Check sheet for the modelled part. Datum: model origin and axes. Units: mm. A direction names the side the tool comes from. Give positions to 0.01 mm unless a question says otherwise; leave off trailing zeros. Order: outer loops, then holes, each group sorted by start corner. A loop starts at its lowest first (then second) coordinate and runs counter-clockwise, first axis right, second up. Notation, with made-up numbers: (-7, 47.25) -> (41, 47.25) arc R24 ccw to (41, 83.25) -> close; hole circle Ø5 at (-33, -30.5). An arc over 180 degrees is marked (long way). One line per question, with ' | ' between items.
```python
from build123d import *

# Parameters (mm, degrees)
IZIM1_W                     = 20
IZIM1_H                     = 20
Y_KSEKLIK_EKSTR_ZYON1_DEPTH = 20
KES_EKSTR_ZYON1_DEPTH       = 20
IZIM3_W                     = 17.224679165
IZIM3_H                     = 17.248412117
KES_EKSTR_ZYON2_DEPTH       = 20
IZIM4_R                     = 2
KES_EKSTR_ZYON3_DEPTH       = 20
IZIM7_R                     = 2.5
KES_EKSTR_ZYON7_DEPTH       = 2
IZIM8_R                     = 2
KES_EKSTR_ZYON8_DEPTH       = 10
IZIM9_R                     = 2.5
KES_EKSTR_ZYON9_DEPTH       = 2


with BuildPart() as part:
    # Çizim1 → Yükseklik-Ekstrüzyon1 (new body)
    with BuildSketch(Plane.XY):
        with Locations((-13.172756411, -5.622082974)):
            Rectangle(IZIM1_W, IZIM1_H)
    extrude(amount=Y_KSEKLIK_EKSTR_ZYON1_DEPTH)

    # Çizim2 → Kes-Ekstrüzyon1 (cut)
    with BuildSketch(Plane.XY.offset(20)):
        Polygon((-3.172756411, 4.377917026), (-23.172756411, -15.622082974), (-23.172756411, 4.377917026), align=None)
    extrude(amount=-KES_EKSTR_ZYON1_DEPTH, mode=Mode.SUBTRACT)

    # Çizim3 → Kes-Ekstrüzyon2 (cut)
    with BuildSketch(Plane.XY.offset(20)):
        with Locations((-15.601705124, -3.767784851)):
            Rectangle(IZIM3_W, IZIM3_H)
    extrude(amount=-KES_EKSTR_ZYON2_DEPTH, mode=Mode.SUBTRACT)

    # Çizim4 → Kes-Ekstrüzyon3 (cut)
    with BuildSketch(Plane.ZY.offset(6.989365541)):
        with Locations((10, -4.007036941)):
            Circle(IZIM4_R)
    extrude(amount=-KES_EKSTR_ZYON3_DEPTH, mode=Mode.SUBTRACT)

    # Çizim7 → Kes-Ekstrüzyon7 (cut)
    with BuildSketch(Plane.ZY.offset(6.989365541)):
        with Locations((10, -4.007036941)):
            Circle(IZIM7_R)
    extrude(amount=-KES_EKSTR_ZYON7_DEPTH, mode=Mode.SUBTRACT)

    # Çizim8 → Kes-Ekstrüzyon8 (cut)
    with BuildSketch(Plane(origin=(0, -12.391990909, 0), x_dir=(1, 0, 0), z_dir=(0, 1, 0))):
        with Locations((-15.081060976, -10)):
            Circle(IZIM8_R)
    extrude(amount=-KES_EKSTR_ZYON8_DEPTH, mode=Mode.SUBTRACT)

    # Çizim9 → Kes-Ekstrüzyon9 (cut)
    with BuildSketch(Plane(origin=(0, -12.391990909, 0), x_dir=(1, 0, 0), z_dir=(0, 1, 0))):
        with Locations((-15.081060976, -10)):
            Circle(IZIM9_R)
    extrude(amount=-KES_EKSTR_ZYON9_DEPTH, mode=Mode.SUBTRACT)


solid = part.part
```
Q1. Mould release check, pull along Y, two halves, no side actions. Record for faces 1 (the face through (-3.173, -8, 10)), 2 (the face through (-4.09, -3.41, 11.91)), 3 (the face through (-4.989, -2, 9)), 4 (the face through (-21.535, -13.984, 10.14)): pulls with the +Y half, pulls with the -Y half, needs draft (parallel to the pull), parting line crosses it, or undercut.
Result sheet:
face 1: needs draft | face 2: undercut | face 3: undercut | face 4: pulls with the +Y half
Q2. Access from +Z, -Z, +X, -X, +Y, -Y to the whole of each face (thin tool, end or side, straight path). Record for faces 5 (the face through (-6, -6.45, 9.46)), 6 (the face through (-16, -14.392, 8)), 7 (the face through (-12, -12.392, 10)), 8 (the face through (-11, -15.622, 10)).
Result sheet:
face 5: -X | face 6: +Y | face 7: +Z, -Z, -X, +Y | face 8: +Z, -Z, +X, -X, -Y
Q3. Section check A-A (z = 10). Enter the section's corners in (x, y), and give its area (3 significant figures).
Result sheet:
outline: (-23.17, -15.62) -> (-17.08, -15.62) -> (-17.08, -14.39) -> (-17.58, -14.39) -> (-17.58, -12.39) -> (-19.94, -12.39) -> close; (-13.08, -15.62) -> (-3.17, -15.62) -> (-3.17, -6.01) -> (-4.99, -6.01) -> (-4.99, -6.51) -> (-6.99, -6.51) -> (-6.99, -12.39) -> (-12.58, -12.39) -> (-12.58, -14.39) -> (-13.08, -14.39) -> close; (-6.99, -1.51) -> (-4.99, -1.51) -> (-4.99, -2.01) -> (-3.17, -2.01) -> (-3.17, 4.38) -> (-6.99, 0.56) -> close | area: 83.9 mm2
Q4. Section check B-B (x = -14.75). Enter the section's corners in (y, z).
Result sheet:
outline: (-15.62, 0) -> (-12.39, 0) -> (-12.39, 7.52) -> (-14.39, 7.52) -> (-14.39, 8.03) -> (-15.62, 8.03) -> close; (-15.62, 11.97) -> (-14.39, 11.97) -> (-14.39, 12.48) -> (-12.39, 12.48) -> (-12.39, 20) -> (-15.62, 20) -> close
Q5. Depth check by flat-ended pin: pin 1 Ø4 at (y, z) = (-3.5, 9) entering from -X; pin 2 Ø12 at (x, z) = (-16, 4) entering from +Y; pin 3 Ø2.5 at (x, z) = (-16, 10) entering from +Y. Enter the tip coordinate at first touch or a pass-through.
Result sheet:
pin 1: stops at x = -6.99 | pin 2: stops at y = -12.39 | pin 3: stops at y = -14.39
Q6. Section check C-C (z = 15). Enter the section's corners in (x, y).
Result sheet:
outline: (-23.17, -15.62) -> (-3.17, -15.62) -> (-3.17, 4.38) -> (-6.99, 0.56) -> (-6.99, -12.39) -> (-19.94, -12.39) -> close
Q7. Thickness scan on line 1 (Z direction, x = -15.25, y = -12.5); line 2 (X direction, y = -1.25, z = 7.25); line 3 (X direction, y = -14.9, z = 10). Record the ranges inside material, lowest first.
Result sheet:
line 1: z = 0 to 7.51, 12.49 to 20 | line 2: x = -6.99 to -3.17 | line 3: x = -22.45 to -17.08, -13.08 to -3.17
Q8. Section check D-D (y = -4.75). Enter the section's corners in (x, z), and give its area (3 significant figures).
Result sheet:
outline: (-6.99, 0) -> (-3.17, 0) -> (-3.17, 8.14) -> (-4.99, 8.14) -> (-4.99, 7.61) -> (-6.99, 7.61) -> close; (-6.99, 12.39) -> (-4.99, 12.39) -> (-4.99, 11.86) -> (-3.17, 11.86) -> (-3.17, 20) -> (-6.99, 20) -> close | area: 60.0 mm2
